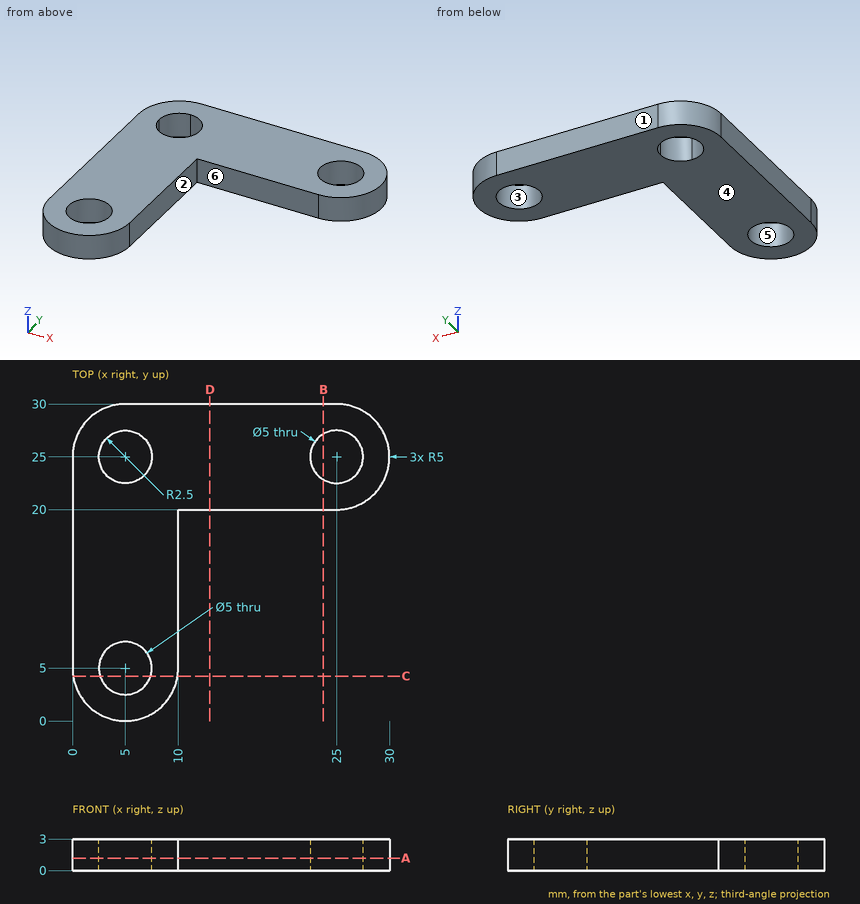
Check sheet for the drawn part. Datum: minimum x, y, z corner. Units: mm. A direction names the side the tool comes from. Round coordinates to 2 decimals unless told otherwise and drop trailing zeros. Order: outer loops, then holes, each group sorted by start corner. A loop starts at its lowest first (then second) coordinate and runs counter-clockwise, first axis right, second up.
1) Mould release check, pull along Y, two halves, no side actions. Record for the marked faces 3, 4, 5 and 6: +Y half, -Y half, draft (parallel to the pull), parting line (faces both ways), or undercut.
2) Tool access check on the marked faces 1 and 2. Record the directions out of +Z, -Z, +X, -X, +Y, -Y that give a thin tool (end or side, any length) a straight path to the whole face; none if there is none.
3) Section check B-B (x = 23.75). Record the boundary of the cut face in (y, z).
4) Section check C-C (y = 4.25). Record the boundary of the cut face in (x, z), and give its area (3 significant figures).
5) Section check A-A (z = 1.2). Record the boundary of the cut face in (x, y), and give its area (3 significant figures).
6) Section check D-D (x = 13). Record the boundary of the cut face in (y, z).
7) Scan lines: line 1 (X direction, y = 27, z = 2.95); line 2 (Y direction, x = 7.25, z = 0.85); line 3 (Y direction, x = 25, z = 1.85). Record each from-to range of solid material in increasing order.
Result:
1. face 3: undercut
1. face 4: draft
1. face 5: undercut
1. face 6: -Y half
2. face 1: +Z, -Z, +X, -X, +Y
2. face 2: +Z, -Z, +X, -Y
3. outline: (20, 0) - (22.83, 0) - (22.83, 3) - (20, 3) - close; (27.17, 0) - (30, 0) - (30, 3) - (27.17, 3) - close
4. outline: (0.06, 0) - (2.62, 0) - (2.62, 3) - (0.06, 3) - close; (7.38, 0) - (9.94, 0) - (9.94, 3) - (7.38, 3) - close
4. area: 15.4 mm2
5. outline: (0, 5) arc R5 ccw to (10, 5) - (10, 20) - (25, 20) arc R5 ccw to (25, 30) - (5, 30) arc R5 ccw to (0, 25) - close; hole circle Ø5 at (5, 5); hole circle Ø5 at (5, 25); hole circle Ø5 at (25, 25)
5. area: 414 mm2
6. outline: (20, 0) - (30, 0) - (30, 3) - (20, 3) - close
7. line 1: x = 0.42 to 3.5, 6.5 to 23.5, 26.5 to 29.58
7. line 2: y = 0.53 to 3.91, 6.09 to 23.91, 26.09 to 30
7. line 3: y = 20 to 22.5, 27.5 to 30
